Job drawing, mm, ordinate dimensions from the low corner. One solid piece. Coordinates: 2 decimals unless noted, no trailing zeros. Order: outer loops, then holes, each group sorted by start corner. A loop starts at its lowest first (then second) coordinate and runs counter-clockwise, first axis right, second up. Notation, with made-up numbers: M 48.25,26.25 L 83.25,26.25 A21 ccw 83.25,51.25 Z; hole C 31,84.5 d9. An arc over 180 degrees is marked long. Write item = value, one per line.
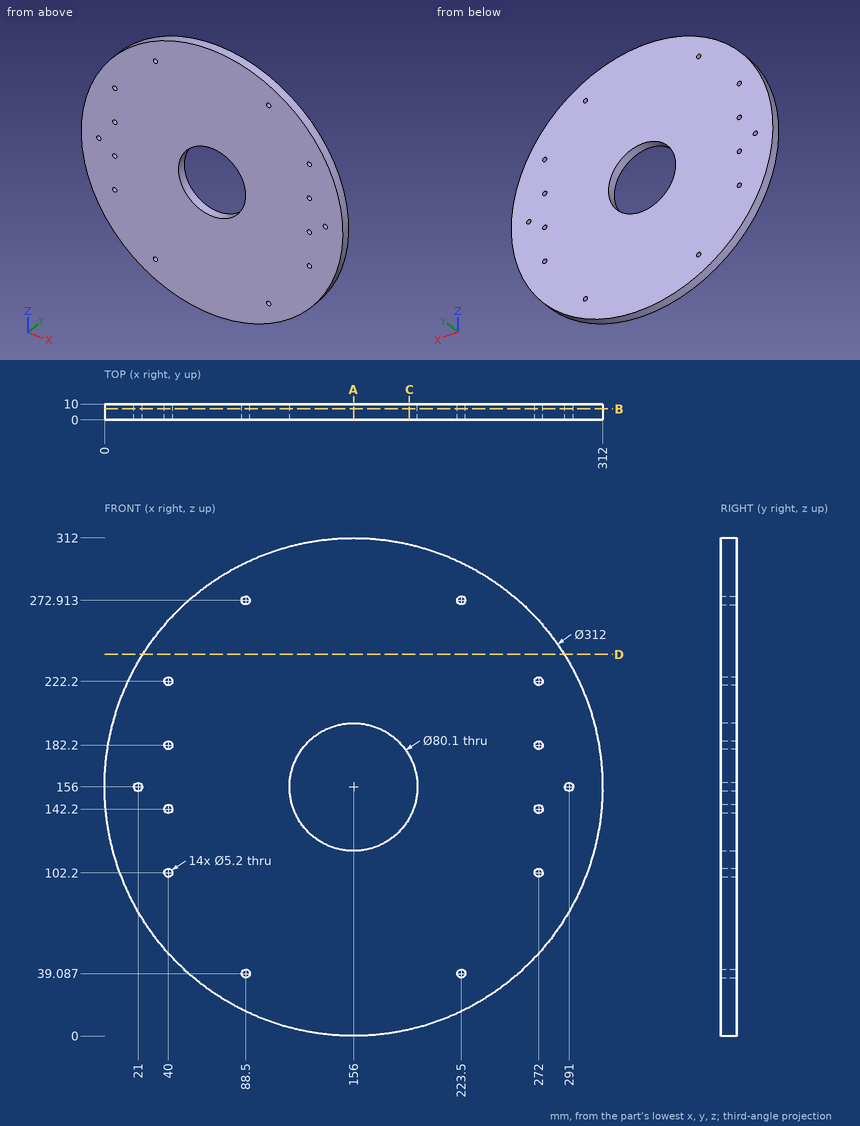
(1) Slice it at C-C, the plane x = 191. Write the cut outline in (y, z).
Evaluation:
outline = M 0,3.98 L 10,3.98 L 10,136.53 L 0,136.53 Z; M 0,175.47 L 10,175.47 L 10,308.02 L 0,308.02 Z
(2) Slice it at A-A, the plane x = 156. Write the cut outline in (y, z), then the cut area to 3 significant figures.
Evaluation:
outline = M 0,0 L 10,0 L 10,115.95 L 0,115.95 Z; M 0,196.05 L 10,196.05 L 10,312 L 0,312 Z
area = 2,320 mm²
(3) Pin check, flat tips, straight feed: pin 1 Ø6 at (y, z) = (8, 74.5) entering from +X; pin 2 Ø1 at (x, y) = (184, 6.5) entering from -Z; pin 3 Ø4.5 at (x, z) = (88.5, 272.91) entering from +Y; pin 4 Ø8.5 at (x, z) = (223.5, 272.91) entering from +Y. Stop position of each tip, or through.
Evaluation:
pin_1 = 290.81
pin_2 = 2.44
pin_3 = through
pin_4 = 10
(4) Slice it at D-D, the plane z = 239. Write the cut outline in (x, y).
Evaluation:
outline = M 23.91,0 L 288.09,0 L 288.09,10 L 23.91,10 Z
(5) Wall check: line 1 (X direction, y = 3.5, z = 156); line 2 (X direction, y = 2.5, z = 182.2) (1 decimal); line 3 (X direction, y = 9, z = 221) (1 decimal). Give the ranges that are in metal, low to high. Write a range as from..to.
Evaluation:
line_1 = 0..18.4, 23.6..115.95, 196.05..288.4, 293.6..312
line_2 = 2.2..37.4, 42.6..125.7, 186.3..269.4, 274.6..309.8
line_3 = 14.2..37.7, 42.3..269.7, 274.3..297.8
(6) Slice it at B-B, the plane y = 7. State how many separate pieces and enclosed holes the cut face has, then the cut area to 3 significant figures.
Evaluation:
separate_pieces = 1
enclosed_holes = 15
area = 71,100 mm²
